Answer from the drawing. Dimensions are ordinates in mm from the lowest x, y and z of the part. A direction names the side the tool comes from. Coordinates: 2 decimals unless noted, no trailing zeros. Order: outer loops, then holes, each group sorted by start corner. A loop starts at its lowest first (then second) coordinate and runs counter-clockwise, first axis right, second up. Notation, with made-up numbers: (-26.5, 47) -> (-16.5, 47) arc R23 cw to (-16.5, 64) -> close; hole circle Ø10 at (-17, 17.25). An arc over 180 degrees is marked (long way). Answer in a Markdown table with one row per item.
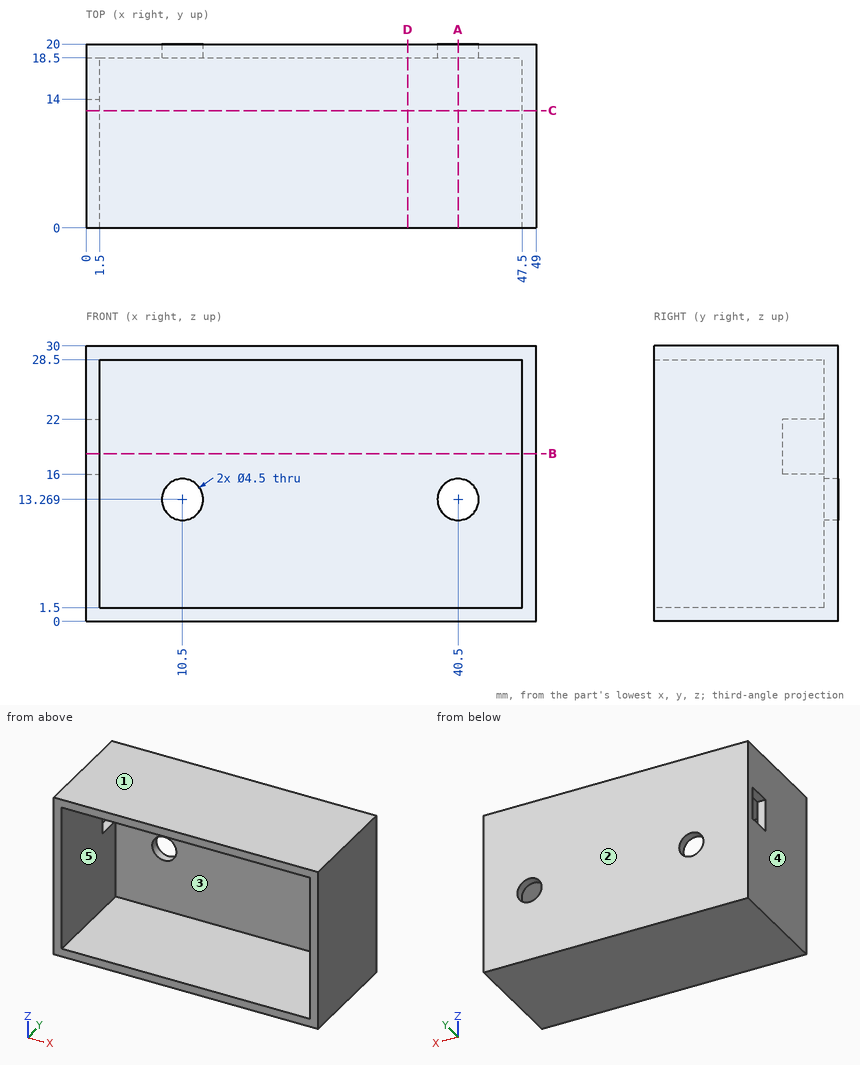
(1) Find the intervals of material crossed by line 1 along Z through (x, y) = (40.5, 19.45); line 2 along X through (y, z) = (10, 5.5); line 3 along Z through (x, y) = (17.5, 7.75), in increasing order. Write a range as from..to.
Check values:
| item | result |
|---|---|
| line 1 | 0..11.02, 15.52..30 |
| line 2 | 0..1.5, 47.5..49 |
| line 3 | 0..1.5, 28.5..30 |
(2) A cutting plane is placed at A-A, the plane x = 40.5. Determine the outline of the cut face in (y, z).
Check values:
| item | result |
|---|---|
| outline | (0, 0) -> (20, 0) -> (20, 11.02) -> (18.5, 11.02) -> (18.5, 1.5) -> (0, 1.5) -> close; (0, 28.5) -> (18.5, 28.5) -> (18.5, 15.52) -> (20, 15.52) -> (20, 30) -> (0, 30) -> close |
(3) A cutting plane is placed at B-B, the plane z = 18.25. Determine the outline of the cut face in (x, y), then the cut area to 3 significant figures.
Check values:
| item | result |
|---|---|
| outline | (0, 0) -> (1.5, 0) -> (1.5, 14) -> (0, 14) -> close; (0, 18.5) -> (47.5, 18.5) -> (47.5, 0) -> (49, 0) -> (49, 20) -> (0, 20) -> close |
| area | 122 mm² |
(4) A flat-ended cylindrical pin translates along its axis: pin 1 (7 mm diameter, centred on x = 40.5, z = 13.27, fed in from -Y). Find the tip coordinate at first contact, or state that the pin passes through.
Check values:
| item | result |
|---|---|
| pin 1 | y = 18.5 |
(5) For a pull along Z with two mould halves and no side action, classify the marked faces 1, 2 and 3 as released by +Z, released by -Z, zero draft, split by the parting line, or undercut.
Check values:
| item | result |
|---|---|
| face 1 | released by +Z |
| face 2 | zero draft |
| face 3 | undercut |
(6) A cutting plane is placed at C-C, the plane y = 12.75. Determine the outline of the cut face in (x, z), then the cut area to 3 significant figures.
Check values:
| item | result |
|---|---|
| outline | (0, 0) -> (49, 0) -> (49, 30) -> (0, 30) -> close; hole (1.5, 1.5) -> (47.5, 1.5) -> (47.5, 28.5) -> (1.5, 28.5) -> close |
| area | 228 mm² |
(7) A cutting plane is placed at D-D, the plane x = 35. Determine the outline of the cut face in (y, z).
Check values:
| item | result |
|---|---|
| outline | (0, 0) -> (20, 0) -> (20, 30) -> (0, 30) -> (0, 28.5) -> (18.5, 28.5) -> (18.5, 1.5) -> (0, 1.5) -> close |
(8) Which of the six approach directions +Z, -Z, +X, -X, +Y, -Y give full straight-line access (tool end or side, diameter ignored) to the marked faces 4 and 5?
Check values:
| item | result |
|---|---|
| face 4 | +Z, -Z, -X, +Y, -Y |
| face 5 | -Y |
